```python
from build123d import *

# Parameters (mm, degrees)
CUT_EXTRUDE1_DEPTH = 5


with BuildPart() as part:
    # Sketch1 → Revolve1 (revolve)
    with BuildSketch(Plane.XY, mode=Mode.PRIVATE) as revolve1_sk:
        Polygon((0, 2), (0, 3), (20.25, 3), (20.25, 4.25), (24.75, 3), (25.5, 3), (25.5, 4.25), (30, 3), (30, 2), align=None)
    revolve(revolve1_sk.sketch.rotate(Axis((0, 0, 0), (1, 0, 0)), 90), axis=Axis((0, 0, 0), (1, 0, 0)))

    # Sketch2 → Cut-Extrude1 (cut, symmetric)
    with BuildSketch(Plane.XY):
        Polygon((0, -3), (6, 3), (0, 3), align=None)
    extrude(amount=CUT_EXTRUDE1_DEPTH, both=True, mode=Mode.SUBTRACT)


solid = part.part
```
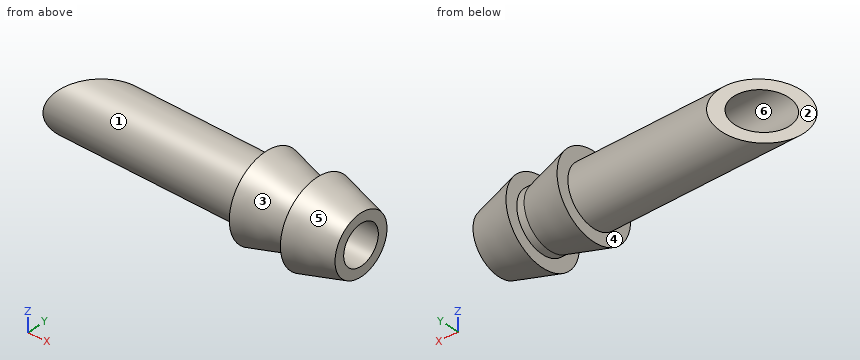
Can you work these out from the model? Positions are in its coordinate system, mm. Face numbers are marked on the shaded views. A direction names the side the tool comes from. Round coordinates to 2 decimals unless told otherwise and drop trailing zeros. Loops run counter-clockwise (first coordinate to the right, second up) from the corner with the lowest first, then second, coordinate; pieces in that order, holes last. Notation, with made-up numbers: M 13,-35 L 49,-35 A15 ccw 49,-12 Z; hole C -25,-3.75 d5. An arc over 180 degrees is marked long. Answer in a Markdown table with one row per item.
1. If we section it at B-B, the plane z = 0: Please give me the cut outline in (x, y), plus the area to 4 significant figures.
Established:
| item | result |
|---|---|
| outline | M 0,-3 L 20.25,-3 L 20.25,-4.25 L 24.75,-3 L 25.5,-3 L 25.5,-4.25 L 30,-3 L 30,-2 L 1,-2 Z; M 5,2 L 30,2 L 30,3 L 25.5,4.25 L 25.5,3 L 24.75,3 L 20.25,4.25 L 20.25,3 L 6,3 Z |
| area | 65.25 mm² |
2. On a 3-axis mill with a long thin cutter (end or side, diameter ignored), from which of +Z, -Z, +X, -X, +Y, -Y can I reach the whole of each face in a straight line? I mean the marked faces 1, 2 and 3. Say none if no direction works.
Established:
| item | result |
|---|---|
| face 1 | -X |
| face 2 | +Z, -Z, -X, +Y |
| face 3 | none |
3. If we section it at D-D, the plane x = 21: Please give me the cut outline in (y, z).
Established:
| item | result |
|---|---|
| outline | C 0,0 d8.08; hole C 0,0 d4 |
4. I'm going to push flat-ended pins straight in: pin 1 Ø1.5 at (y, z) = (2, 1) entering from -X; pin 2 Ø3 at (x, z) = (3.5, 0.5) entering from -Y; pin 3 Ø2.5 at (y, z) = (-1, -1.5) entering from -X. Where does each tip first touch, or does it pass through?
Established:
| item | result |
|---|---|
| pin 1 | x = 4.39 |
| pin 2 | y = -3 |
| pin 3 | x = 0.75 |
5. Please list where these lines run through material, in increasing order: line 1 (Y direction, x = 10.5, z = 0); line 2 (Z direction, x = 11.5, y = 1.75); line 3 (Z direction, x = 7.5, y = -0.25). Write a range as from..to.
Established:
| item | result |
|---|---|
| line 1 | -3..-2, 2..3 |
| line 2 | -2.44..-0.97, 0.97..2.44 |
| line 3 | -2.99..-1.98, 1.98..2.99 |
6. If we section it at A-A, the plane y = 0: Please give me the cut outline in (x, z), plus the area to 4 significant figures.
Established:
| item | result |
|---|---|
| outline | M 3,-3 L 20.25,-3 L 20.25,-4.25 L 24.75,-3 L 25.5,-3 L 25.5,-4.25 L 30,-3 L 30,-2 L 3,-2 Z; M 3,2 L 30,2 L 30,3 L 25.5,4.25 L 25.5,3 L 24.75,3 L 20.25,4.25 L 20.25,3 L 3,3 Z |
| area | 65.25 mm² |
7. If we section it at C-C, the plane x = 8: Please give me the cut outline in (y, z), plus the area to 3 significant figures.
Established:
| item | result |
|---|---|
| outline | C 0,0 d6; hole C 0,0 d4 |
| area | 15.7 mm² |
8. Thinking about a two-plate mould opening in Z: for the marked faces 4, 5 and 6, which applies, pulls with the +Z half, pulls with the -Z half, needs draft (parallel to the pull), parting line crosses it, or undercut?
Established:
| item | result |
|---|---|
| face 4 | needs draft |
| face 5 | parting line crosses it |
| face 6 | undercut |
